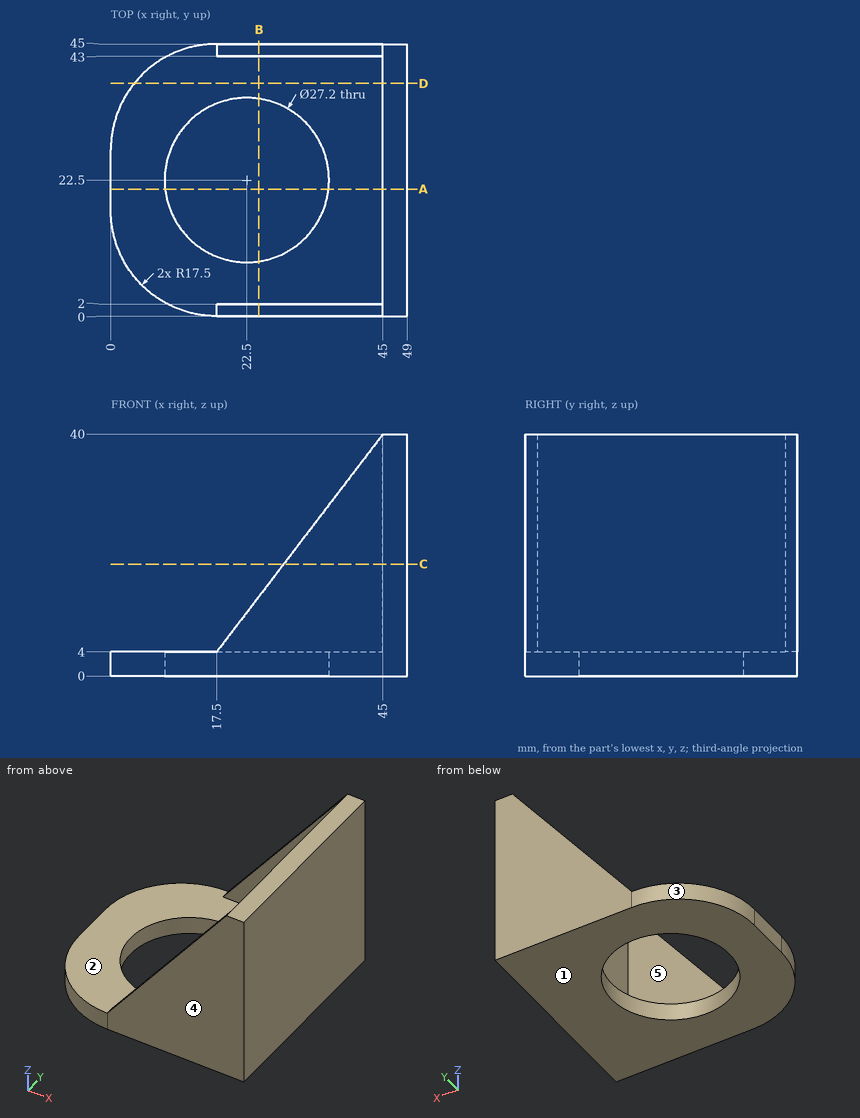
Part print with two shaded views. Sizes in mm from the minimum x, y, z corner. A direction names the side the tool comes from. Round coordinates to 2 decimals unless told otherwise and drop trailing zeros. Loops run counter-clockwise (first coordinate to the right, second up) from the corner with the lowest first, then second, coordinate; pieces in that order, holes last.
Item 1: Drill centre lines: line 1 along Y through (x, z) = (22, 3); line 2 along X through (y, z) = (22, 3); line 3 along Z through (x, y) = (11.5, 14). Where is each one in solid material? Low to high.
Item 2: Saw through at B-B (x = 24.5). List the corners of the cut face in (y, z), then the cut area to 3 significant figures.
Item 3: Two-plate mould, pull along Y, no slides. Class the marked faces 3, 4 and 5: released by +Y, released by -Y, zero draft, split by the parting line, or undercut.
Item 4: Which spindle directions (+Z, -Z, +X, -X, +Y, -Y) get a long thin tool onto all of the face, cutting with end or side? Do the marked faces 1 and 2. Say none if no direction does.
Item 5: Pin check, flat tips, straight feed: P1, Ø1, axis at y = 15.5, z = 22.5, coming from the -X side; P2, Ø13.5, axis at x = 28, y = 30.5, coming from the +Z side; P3, Ø1.5, axis at x = 24, y = 10, coming from the -Z side. Stop position of each tip, or through.
Item 6: Saw through at A-A (y = 21). List the corners of the cut face in (x, z).
Item 7: Saw through at D-D (y = 38.5). List the corners of the cut face in (x, z).
Item 8: Saw through at C-C (z = 18.5). List the corners of the cut face in (x, y), then the cut area to 3 significant figures.
Worked answers:
1. line 1: y = 0 to 8.91, 36.09 to 45
1. line 2: x = 0 to 8.91, 36.09 to 49
1. line 3: z = 0 to 4
2. outline: (0, 0) - (9.05, 0) - (9.05, 4) - (2, 4) - (2, 13.16) - (0, 13.16) - close; (35.95, 0) - (45, 0) - (45, 13.16) - (43, 13.16) - (43, 4) - (35.95, 4) - close
2. area: 109 mm2
3. face 3: released by +Y
3. face 4: released by -Y
3. face 5: undercut
4. face 1: -Z, +X, -X, +Y, -Y
4. face 2: +Z, -X
5. P1: stops at x = 45
5. P2: stops at z = 4
5. P3: passes through
6. outline: (0, 0) - (8.98, 0) - (8.98, 4) - (0, 4) - close; (36.02, 0) - (49, 0) - (49, 40) - (45, 40) - (45, 4) - (36.02, 4) - close
7. outline: (3.89, 0) - (49, 0) - (49, 40) - (45, 40) - (45, 4) - (3.89, 4) - close
8. outline: (28.58, 0) - (49, 0) - (49, 45) - (28.58, 45) - (28.58, 43) - (45, 43) - (45, 2) - (28.58, 2) - close
8. area: 246 mm2
